from build123d import *

# Parameters (mm, degrees)
SKETCH1_R           = 370
BOSS_EXTRUDE1_DEPTH = 1
CUT_EXTRUDE1_REACH  = 525.263
SKETCH2_R           = 4.5


with BuildPart() as part:
    # Sketch1 → Boss-Extrude1 (new, symmetric)
    with BuildSketch(Plane(origin=(0, 0, 0), x_dir=(1, 0, 0), z_dir=(0, 1, 0))):
        with Locations(Location((0, 0, 0), (0, 0, 270))):
            Circle(SKETCH1_R)
    extrude(amount=BOSS_EXTRUDE1_DEPTH, both=True)

    # Sketch2 → Cut-Extrude1 (cut, up to next)
    with BuildSketch(Plane(origin=(0, 1, 0), x_dir=(1, 0, 0), z_dir=(0, 1, 0)), mode=Mode.PRIVATE) as cut_extrude1_sk1:
        with Locations(Location((0, -351.5, 0), (0, 0, 270))):
            Circle(SKETCH2_R)
    cut_extrude1_tool1 = extrude(cut_extrude1_sk1.sketch, amount=-CUT_EXTRUDE1_REACH, mode=Mode.PRIVATE) & part.part
    # Sketch2 → Cut-Extrude1 (cut, up to next)
    with BuildSketch(Plane(origin=(0, 1, 0), x_dir=(1, 0, 0), z_dir=(0, 1, 0)), mode=Mode.PRIVATE) as cut_extrude1_sk2:
        with Locations(Location((0, -326.5, 0), (0, 0, 270))):
            Circle(SKETCH2_R)
    cut_extrude1_tool2 = extrude(cut_extrude1_sk2.sketch, amount=-CUT_EXTRUDE1_REACH, mode=Mode.PRIVATE) & part.part
    # Sketch2 → Cut-Extrude1 (cut, up to next)
    with BuildSketch(Plane(origin=(0, 1, 0), x_dir=(1, 0, 0), z_dir=(0, 1, 0)), mode=Mode.PRIVATE) as cut_extrude1_sk3:
        with Locations(Location((0, 326.5, 0), (0, 0, 270))):
            Circle(SKETCH2_R)
    cut_extrude1_tool3 = extrude(cut_extrude1_sk3.sketch, amount=-CUT_EXTRUDE1_REACH, mode=Mode.PRIVATE) & part.part
    # Sketch2 → Cut-Extrude1 (cut, up to next)
    with BuildSketch(Plane(origin=(0, 1, 0), x_dir=(1, 0, 0), z_dir=(0, 1, 0)), mode=Mode.PRIVATE) as cut_extrude1_sk4:
        with Locations(Location((0, 351.5, 0), (0, 0, 270))):
            Circle(SKETCH2_R)
    cut_extrude1_tool4 = extrude(cut_extrude1_sk4.sketch, amount=-CUT_EXTRUDE1_REACH, mode=Mode.PRIVATE) & part.part
    add(cut_extrude1_tool1.solids().sort_by_distance((0, 1, 351.5))[0], mode=Mode.SUBTRACT)
    add(cut_extrude1_tool2.solids().sort_by_distance((0, 1, 326.5))[0], mode=Mode.SUBTRACT)
    add(cut_extrude1_tool3.solids().sort_by_distance((0, 1, -326.5))[0], mode=Mode.SUBTRACT)
    add(cut_extrude1_tool4.solids().sort_by_distance((0, 1, -351.5))[0], mode=Mode.SUBTRACT)


solid = part.part
Read the model definition and answer for the solid it produces. Units are mm, in the model's axes. Give positions to 0.01 mm unless a question says otherwise; leave off trailing zeros. Write each loop counter-clockwise with the first axis right and the second up, starting at its lowest first coordinate (ties: lowest second). Pieces come first, ordered by that corner, then holes. Notation, with made-up numbers: (-2, 64) - (57, 64) arc R27 cw to (57, 83) - close; hole circle Ø7 at (19, 64). An arc over 180 degrees is marked (long way). Return JSON: item names as keys, results as strings.
Q1. Consider line 1 along X through (y, z) = (-0.4, 326.5); line 2 along X through (y, z) = (0.2, 5.5); line 3 along Z through (x, y) = (-42, -0.9). Determine where each line is inside the solid, lowest interval first. Write a range as [from, to].
Reply:
{"line 1": "[-174.06, -4.5], [4.5, 174.06]", "line 2": "[-369.96, 369.96]", "line 3": "[-367.61, 367.61]"}
Q2. Given P1, Ø8, axis at x = 0, z = -326.5, coming from the +Y side, flat-ended and moving along its own axis, determine where the tip first touches the part or whether it passes through.
Reply:
{"P1": "through"}
Q3. A cutting plane is placed at A-A, the plane y = -0.2. Determine the outline of the cut face in (x, z), and give its area (3 significant figures).
Reply:
{"outline": "circle Ø740 at (0, 0); hole circle Ø9 at (0, -351.5); hole circle Ø9 at (0, -326.5); hole circle Ø9 at (0, 326.5); hole circle Ø9 at (0, 351.5)", "area": "430,000 mm²"}
Q4. A cutting plane is placed at B-B, the plane x = 262. Determine the outline of the cut face in (y, z), and give its area (3 significant figures).
Reply:
{"outline": "(-1, -261.26) - (1, -261.26) - (1, 261.26) - (-1, 261.26) - close", "area": "1,050 mm²"}
Q5. A cutting plane is placed at C-C, the plane z = -69.5. Determine the outline of the cut face in (x, y), and give its area (3 significant figures).
Reply:
{"outline": "(-363.41, -1) - (363.41, -1) - (363.41, 1) - (-363.41, 1) - close", "area": "1,450 mm²"}
